For this review, take the finished solid that the model builds, in its own axes (mm). A direction names the side the tool comes from. Give positions to 0.01 mm unless a question says otherwise; leave off trailing zeros. Order: outer loops, then holes, each group sorted by start corner. A loop starts at its lowest first (then second) coordinate and runs counter-clockwise, first axis right, second up. Notation, with made-up numbers: (15, 70) - (48, 70) arc R18 ccw to (48, 79) - close; hole circle Ø6 at (54, 21). An arc over 180 degrees is marked (long way). Use a Markdown table: item, result. Add a question column.
1) Mouldability with a two-part tool opening along X and no side actions: class faces 1 (the face through (-15.497, 1.107, -59.303)), 2 (the face through (-35.185, 9, -30)), 3 (the face through (-6, 0, -31)) as released by +X, released by -X, zero draft, split by the parting line, or undercut.
2) We need section B-B on y = 11.25. Write out the cut boundary in (x, z).
3) We need section A-A on z = -49. Write out the cut boundary in (x, y).
4) We need section D-D on x = -25. Write out the cut boundary in (y, z).
5) Clearance check with flat-ended pins moving along their axes: P1, Ø5, axis at x = -50.5, y = 9.5, coming from the -Z side; P2, Ø1.5, axis at x = -11, z = -19.5, coming from the +Y side; P3, Ø3.5, axis at y = 8.71, z = -46.48, coming from the +X side. State where each tip first meets the part, or that it passes through.
6) Wall thickness on L1, parallel to Y at x = 0, z = -14.5; L2, parallel to X at y = 1.5, z = -20.5; L3, parallel to X at y = 5.5, z = -42: over which ranges is each line inside the solid? List them lowest first.
7) We need section C-C on x = -16. Write out the cut boundary in (y, z), then the cut area to 3 significant figures.
8) Machinability: for faces 4 (the face through (-15.4, 1.1, -1.9)), 5 (the face through (-15.318, 3.472, -0.377)), 6 (the face through (-28.39, 8.19, -13.48)), 7 (the face through (-9.455, 9, -30)), which of the approach directions +Z, -Z, +X, -X, +Y, -Y give a long, thin tool a straight path to every point of the face, cutting with its end or side? Answer none if there is none.
```python
from build123d import *

# Parameters (mm, degrees)
SKETCH1_W             = 88.138
SKETCH1_H             = 101.6
BOSS_EXTRUDE1_DEPTH   = 12.7
SKETCH2_W             = 24.3078
SKETCH2_H             = 101.6
SKETCH2_W_2           = 11.938
CUT_EXTRUDE1_DEPTH    = 7.9756
CUT_EXTRUDE2_DEPTH    = 102.139918983
CUT_EXTRUDE3_DEPTH    = 2.54
F_6_32_TAPPED_HOLE1_D = 2.7051
FILLET1_R             = 3.175
CUT_EXTRUDE4_DEPTH    = 105.220067893


with BuildPart() as part:
    # Sketch1 → Boss-Extrude1 (new body)
    with BuildSketch(Plane(origin=(0, 0, 0), x_dir=(1, 0, 0), z_dir=(0, 1, 0))):
        with Locations((-15.42415, 30.601708333)):
            Rectangle(SKETCH1_W, SKETCH1_H)
    extrude(amount=BOSS_EXTRUDE1_DEPTH)

    # Sketch2 → Cut-Extrude1 (cut)
    with BuildSketch(Plane(origin=(0, 12.7, 0), x_dir=(1, 0, 0), z_dir=(0, 1, 0))):
        with Locations((-47.33925, 30.601708333)):
            Rectangle(SKETCH2_W, SKETCH2_H)
        with Locations((16.49095, 30.601708333)):
            Rectangle(SKETCH2_W, SKETCH2_H)
        with Locations((-15.42415, 30.601708333)):
            Rectangle(SKETCH2_W_2, SKETCH2_H)
    extrude(amount=-CUT_EXTRUDE1_DEPTH, mode=Mode.SUBTRACT)

    # Sketch3 → Cut-Extrude2 (cut, through all)
    with BuildSketch(Plane(origin=(0, 4.7244, 0), x_dir=(1, 0, 0), z_dir=(0, 1, 0))):
        with BuildLine():
            Line((-18.72615, 5.201708333), (-18.72615, 56.001708333))
            ThreePointArc((-18.72615, 56.001708333), (-15.42415, 59.303708333), (-12.12215, 56.001708333))
            Line((-12.12215, 56.001708333), (-12.12215, 5.201708333))
            ThreePointArc((-12.12215, 5.201708333), (-15.42415, 1.899708333), (-18.72615, 5.201708333))
        make_face()
    extrude(amount=-CUT_EXTRUDE2_DEPTH, mode=Mode.SUBTRACT)

    # Sketch4 → Cut-Extrude3 (cut)
    with BuildSketch(Plane(origin=(0, 4.7244, 0), x_dir=(1, 0, 0), z_dir=(0, 1, 0))):
        with BuildLine():
            Line((-20.25015, 5.201708333), (-20.25015, 56.001708333))
            ThreePointArc((-20.25015, 56.001708333), (-15.42415, 60.827708333), (-10.59815, 56.001708333))
            Line((-10.59815, 56.001708333), (-10.59815, 5.201708333))
            ThreePointArc((-10.59815, 5.201708333), (-15.42415, 0.375708333), (-20.25015, 5.201708333))
        make_face()
    extrude(amount=-CUT_EXTRUDE3_DEPTH, mode=Mode.SUBTRACT)

    # #6-32 Tapped Hole1 (through all)
    with Locations(Plane(origin=(4.33705, 0, 0), x_dir=(0, 0, -1), z_dir=(1, 0, 0))):
        with Locations((14.726708333, 8.7122), (46.476708333, 8.7122)):
            Hole(F_6_32_TAPPED_HOLE1_D / 2)

    # Fillet1
    fillet1_edges = [part.edges().sort_by_distance(p)[0] for p in [
        (-59.49315, 2.3622, -81.401708333),
        (-59.49315, 2.3622, 20.198291667),
        (28.64485, 2.3622, -81.401708333),
        (28.64485, 2.3622, 20.198291667),
    ]]
    fillet(fillet1_edges, radius=FILLET1_R)

    # Sketch8 → Cut-Extrude4 (cut, through all)
    with BuildSketch(Plane.ZY.offset(35.18535)):
        Polygon((-6.128808333, 4.7244), (-9.206801398, 12.7762), (20.198291667, 12.7), (20.198291667, 4.7244), align=None)
        Polygon((-55.074608333, 4.7244), (-51.996615269, 12.7762), (-81.401708333, 12.7), (-81.401708333, 4.7244), align=None)
    extrude(amount=-CUT_EXTRUDE4_DEPTH, mode=Mode.SUBTRACT)


solid = part.part
```
Checked values:
| question | item | result |
|---|---|---|
| 1 | face 1 | undercut |
| 1 | face 2 | released by -X |
| 1 | face 3 | zero draft |
| 2 | outline | (-35.19, -52.58) - (-21.39, -52.58) - (-21.39, -8.62) - (-35.19, -8.62) - close; (-9.46, -52.58) - (4.34, -52.58) - (4.34, -8.62) - (-9.46, -8.62) - close |
| 3 | outline | (-59.49, 0) - (-18.73, 0) - (-18.73, 2.18) - (-20.25, 2.18) - (-20.25, 4.72) - (-21.39, 4.72) - (-21.39, 12.7) - (-35.19, 12.7) - (-35.19, 4.72) - (-59.49, 4.72) - close; (-12.12, 0) - (28.64, 0) - (28.64, 4.72) - (4.34, 4.72) - (4.34, 12.7) - (-9.46, 12.7) - (-9.46, 4.72) - (-10.6, 4.72) - (-10.6, 2.18) - (-12.12, 2.18) - close |
| 4 | outline | (0, -81.4) - (4.72, -81.4) - (4.72, -55.07) - (12.7, -52.03) - (12.7, -9.18) - (4.72, -6.13) - (4.72, 20.2) - (0, 20.2) - close; hole circle Ø2.71 at (8.71, -46.48); hole circle Ø2.71 at (8.71, -14.73) |
| 5 | P1 | through |
| 5 | P2 | y = 4.72 |
| 5 | P3 | x = 4.34 |
| 6 | L1 | 0 to 7.38, 10.05 to 12.7 |
| 6 | L2 | -59.49 to -18.73, -12.12 to 28.64 |
| 6 | L3 | -35.19 to -21.39, -9.46 to 4.34 |
| 7 | outline | (0, -81.4) - (4.72, -81.4) - (4.72, -60.79) - (2.18, -60.79) - (2.18, -59.25) - (0, -59.25) - close; (0, -1.95) - (2.18, -1.95) - (2.18, -0.41) - (4.72, -0.41) - (4.72, 20.2) - (0, 20.2) - close |
| 7 | area | 201 mm² |
| 8 | face 4 | +Y, -Y |
| 8 | face 5 | +Y |
| 8 | face 6 | +X, -X |
| 8 | face 7 | +Z, -Z, +Y |
